```python
from build123d import *

# Parameters (mm, degrees)
SKETCH2_W           = 120
SKETCH2_H           = 120
BOSS_EXTRUDE1_DEPTH = 50
SKETCH3_R           = 35
BOSS_EXTRUDE2_DEPTH = 25
SKETCH4_R           = 25
CUT_EXTRUDE1_DEPTH  = 76
FILLET2_R           = 1.5
FILLET7_R           = 10
FILLET8_R           = 5
SHELL1_T            = -2


with BuildPart() as part:
    # Sketch2 → Boss-Extrude1 (new body)
    with BuildSketch(Plane.XY):
        Rectangle(SKETCH2_W, SKETCH2_H)
    extrude(amount=BOSS_EXTRUDE1_DEPTH)

    # Sketch3 → Boss-Extrude2 (add)
    with BuildSketch(Plane(origin=(0, 0, 0), x_dir=(-1, 0, 0), z_dir=(0, 0, -1))):
        Circle(SKETCH3_R)
    extrude(amount=BOSS_EXTRUDE2_DEPTH)

    # Sketch4 → Cut-Extrude1 (cut, through all)
    with BuildSketch(Plane(origin=(0, 0, -25), x_dir=(-1, 0, 0), z_dir=(0, 0, -1))):
        Circle(SKETCH4_R)
    extrude(amount=-CUT_EXTRUDE1_DEPTH, mode=Mode.SUBTRACT)

    # Fillet2
    fillet2_edges = [part.edges().sort_by_distance(p)[0] for p in [
        (35, 0, -25),
        (25, 0, -25),
    ]]
    fillet(fillet2_edges, radius=FILLET2_R)

    # Fillet7
    fillet7_edges = [part.edges().sort_by_distance(p)[0] for p in [
        (-60, 60, 25),
        (60, 60, 25),
        (60, -60, 25),
        (-60, -60, 25),
    ]]
    fillet(fillet7_edges, radius=FILLET7_R)

    # Fillet8
    fillet8_edges = [part.edges().sort_by_distance(p)[0] for p in [
        (0, -60, 0),
        (-60, 0, 0),
        (0, 60, 0),
        (60, 0, 0),
        (57.071067812, 57.071067812, 0),
        (-57.071067812, 57.071067812, 0),
        (57.071067812, -57.071067812, 0),
        (-57.071067812, -57.071067812, 0),
    ]]
    fillet(fillet8_edges, radius=FILLET8_R)

    # Shell1
    shell1_openings = [part.faces().sort_by_distance(p)[0] for p in [
        (-25, 0, 50),
    ]]
    offset(amount=SHELL1_T, openings=shell1_openings, kind=Kind.INTERSECTION)


solid = part.part
```
Here's how the part is built. I have some questions about the finished solid (model axes, mm). A direction names the side the tool comes from. Coordinates: 2 decimals unless noted, no trailing zeros. Write each loop counter-clockwise with the first axis right and the second up, starting at its lowest first coordinate (ties: lowest second). Pieces come first, ordered by that corner, then holes. Notation, with made-up numbers: (-9, 85) -> (38, 85) arc R35 cw to (38, 119) -> close; hole circle Ø11 at (53, 2.25). An arc over 180 degrees is marked (long way). Use a Markdown table: item, result. Add a question column.
(1) For faces 1 (the cylindrical face through (5.85, -26.36, 12.99)), 2 (the flat face through (24, -8, 50)), which set-ups out of +Z, -Z, +X, -X, +Y, -Y let a thin tool reach every point of the face, with its end or its side?
(2) We'd pull the mould along X, two halves only. Please class faces 3 (the cylindrical face through (-57.15, 56.99, 27.82)), 4 (the cylindrical face through (56.99, 57.15, 27.82)), 5 (the flat face through (-58, -1, 27)): +X half, -X half, draft (parallel to the pull), parting line (faces both ways), or undercut.
(3) I'm going to push flat-ended pins straight in: P1, Ø4, axis at x = -36, y = 35, coming from the -Z side; P2, Ø4, axis at y = 13, z = -17.5, coming from the -X side; P3, Ø10, axis at y = -12.5, z = -6.5, coming from the +X side. Where does each tip first touch, or does it pass through?
(4) If we section it at A-A, the plane z = 10: Write out the boundary of the cut face in (x, y), and give its area (3 significant figures).
(5) If we section it at D-D, the plane x = -39.5: Write out the boundary of the cut face in (y, z), and give its area (3 significant figures).
(6) Please list where these lines run through material, in increasing order: line 1 (Y direction, x = 0, z = -0.5); line 2 (X direction, y = -0.5, z = -6) (3 decimals); line 3 (X direction, y = -47, z = 35).
Outcome:
| question | item | result |
|---|---|---|
| 1 | face 1 | +Z |
| 1 | face 2 | +Z, +X, -X, +Y, -Y |
| 2 | face 3 | -X half |
| 2 | face 4 | +X half |
| 2 | face 5 | undercut |
| 3 | P1 | stops at z = 0 |
| 3 | P2 | stops at x = -33.23 |
| 3 | P3 | stops at x = 34.19 |
| 4 | outline | (-60, -50) arc R10 ccw to (-50, -60) -> (50, -60) arc R10 ccw to (60, -50) -> (60, 50) arc R10 ccw to (50, 60) -> (-50, 60) arc R10 ccw to (-60, 50) -> close; circle Ø54 at (0, 0); hole (-58, -50) arc R8 ccw to (-50, -58) -> (50, -58) arc R8 ccw to (58, -50) -> (58, 50) arc R8 ccw to (50, 58) -> (-50, 58) arc R8 ccw to (-58, 50) -> close; hole circle Ø50 at (0, 0) |
| 4 | area | 1,240 mm^2 |
| 5 | outline | (-60, 5) arc R5 ccw to (-55, 0) -> (55, 0) arc R5 ccw to (60, 5) -> (60, 50) -> (58, 50) -> (58, 5) arc R3 cw to (55, 2) -> (-55, 2) arc R3 cw to (-58, 5) -> (-58, 50) -> (-60, 50) -> close |
| 5 | area | 425 mm^2 |
| 6 | line 1 | y = -35 to -33, -27 to -25, 25 to 27, 33 to 35 |
| 6 | line 2 | x = -34.996 to -32.996, -26.995 to -24.995, 24.995 to 26.995, 32.996 to 34.996 |
| 6 | line 3 | x = -60 to -58, 58 to 60 |
